Could you check a few things on this drawing? It's one solid part, dimensions in mm from its lowest x, y, z. A direction names the side the tool comes from. Give positions to 0.01 mm unless a question says otherwise; leave off trailing zeros. Order: outer loops, then holes, each group sorted by start corner. A loop starts at its lowest first (then second) coordinate and runs counter-clockwise, first axis right, second up. Notation, with made-up numbers: (39, 72) -> (75, 72) arc R18 cw to (75, 76) -> close; hole circle Ø1 at (74.5, 7.25). An arc over 180 degrees is marked (long way). Write each question's results on one line, items separated by ' | '.
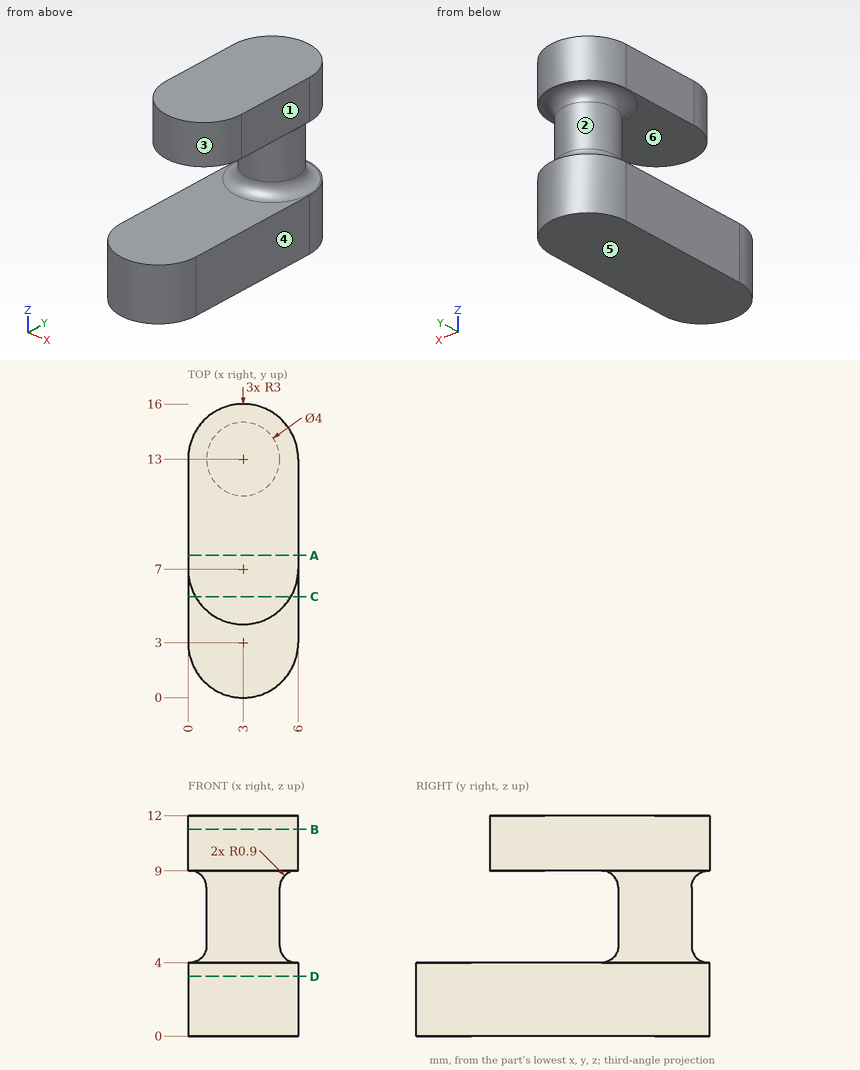
Q1. Suppose I cut it at B-B on z = 11.25. Please give me the cut outline in (x, y).
Here are the results:
outline: (0, 7) arc R3 ccw to (6, 7) -> (6, 13) arc R3 ccw to (0, 13) -> close
Q2. I'm going to push flat-ended pins straight in: pin 1 Ø1.5 at (x, z) = (0.5, 1.5) entering from -Y; pin 2 Ø1.5 at (x, z) = (4.5, 10) entering from +Y. Where does each tip first touch, or does it pass through?
Here are the results:
pin 1: stops at y = 0.56 | pin 2: stops at y = 15.9
Q3. Suppose I cut it at A-A on y = 7.75. Please give me the cut outline in (x, z), and give its area (3 significant figures).
Here are the results:
outline: (0, 0) -> (6, 0) -> (6, 4) -> (0, 4) -> close; (0, 9) -> (6, 9) -> (6, 12) -> (0, 12) -> close | area: 42.0 mm²
Q4. I need wall thicknesses on line 1 along Z through (x, y) = (1.3, 5.5); line 2 along Z through (x, y) = (5.55, 2); line 3 along Y through (x, z) = (3.55, 11). Which ranges of each line are inside material? Lowest first, please.
Here are the results:
line 1: z = 0 to 4, 9 to 12 | line 2: z = 0 to 4 | line 3: y = 4.05 to 15.95
Q5. For the marked faces 1, 2 and 3, which set-ups out of +Z, -Z, +X, -X, +Y, -Y let a thin tool reach every point of the face, with its end or its side?
Here are the results:
face 1: +Z, -Z, +X, +Y, -Y | face 2: none | face 3: +Z, -Y
Q6. Suppose I cut it at C-C on y = 5.5. Please give me the cut outline in (x, z).
Here are the results:
outline: (0, 0) -> (6, 0) -> (6, 4) -> (0, 4) -> close; (0.4, 9) -> (5.6, 9) -> (5.6, 12) -> (0.4, 12) -> close
Q7. Suppose I cut it at D-D on z = 3.25. Please give me the cut outline in (x, y).
Here are the results:
outline: (0, 3) arc R3 ccw to (6, 3) -> (6, 13) arc R3 ccw to (0, 13) -> close
Q8. Thinking about a two-plate mould opening in Z: for the marked faces 4, 5 and 6, which applies, +Z half, -Z half, draft (parallel to the pull), parting line (faces both ways), or undercut?
Here are the results:
face 4: draft | face 5: -Z half | face 6: undercut
